Verification items for the finished model (mm, model axes). Face numbers are marked on the shaded views. A direction names the side the tool comes from. Give positions to 0.01 mm unless a question says otherwise; leave off trailing zeros. Loops run counter-clockwise (first coordinate to the right, second up) from the corner with the lowest first, then second, coordinate; pieces in that order, holes last. Notation, with made-up numbers: (-4, 46.5) -> (40, 46.5) arc R21 cw to (40, 60.5) -> close; hole circle Ø4 at (73.5, -23.5). An arc over 180 degrees is marked (long way). Answer in a Markdown table with one row per item. Add a question column.
Q1. Material ranges on probe 1 along Y at (x, z) = (0, 5.3); probe 2 along Y at (x, z) = (-3, -11); probe 3 along Z at (x, y) = (-44.5, 37.5), recorded low to high.
Q2. Gauge pin test, flat ends, axial feed: P1, Ø1, axis at x = -36, z = -14.5, coming from the -Y side; P2, Ø0.6, axis at y = 0.5, z = 5, coming from the +X side; P3, Ø2, axis at x = -12.5, y = -20, coming from the +Z side. Record the tip position at first contact, or that the pin passes through.
Q3. Section check A-A on y = -27.5. Enter the section's corners in (x, z), and give its area (3 significant figures).
Q4. Section check D-D on z = -3.25. Enter the section's corners in (x, y), and give its area (3 significant figures).
Q5. Set-up check for the marked faces 5, 6 and 7: record each of +Z, -Z, +X, -X, +Y, -Y from which the full face is reachable in a straight line by a thin tool's end or side.
Q6. Section check C-C on y = -6. Enter the section's corners in (x, z).
Q7. Release check for a two-part mould opening along Z. For the marked faces 1, 2, 3 and 4 record: pulls with the +Z half, pulls with the -Z half, needs draft (parallel to the pull), parting line crosses it, or undercut.
Q8. Section check B-B on x = -15. Enter the section's corners in (y, z), and give its area (3 significant figures).
```python
from build123d import *

# Parameters (mm, degrees)
EXTRUDE_1_DEPTH     = 4
SKETCH_2_R          = 5
EXTRUDE_2_DEPTH     = 2
SKETCH_3_W          = 0.972791726
SKETCH_3_H          = 7.511993454
EXTRUDE_3_DEPTH     = 2
CUT_EXTRUDE_1_DEPTH = 2
FILLET_1_R          = 2
SKETCH_5_W          = 26
SKETCH_5_H          = 116
EXTRUDE_4_DEPTH     = 14
EXTRUDE_5_DEPTH     = 2


with BuildPart() as part:
    # 草图1 → 凸台-拉伸1 (new body)
    with BuildSketch(Plane.XY):
        with BuildLine():
            Line((-16.5, -55.5), (-16.5, 55.5))
            ThreePointArc((-16.5, 55.5), (0, 72), (16.5, 55.5))
            Line((16.5, 55.5), (16.5, -55.5))
            ThreePointArc((16.5, -55.5), (0, -72), (-16.5, -55.5))
        make_face()
    extrude(amount=EXTRUDE_1_DEPTH)

    # 草图2 → 凸台-拉伸2 (add)
    with BuildSketch(Plane.XY.offset(4)):
        with BuildLine():
            Line((-8.5, -37.5), (-8.5, 37.5))
            ThreePointArc((-8.5, 37.5), (0, 46), (8.5, 37.5))
            Line((8.5, 37.5), (8.5, -37.5))
            ThreePointArc((8.5, -37.5), (0, -46), (-8.5, -37.5))
        make_face()
        with Locations((0, -27.5)):
            Circle(SKETCH_2_R, mode=Mode.SUBTRACT)
    extrude(amount=EXTRUDE_2_DEPTH)

    # 草图3 → 凸台-拉伸3 (add)
    with BuildSketch(Plane.XY.offset(4)):
        with Locations((0, -27.5)):
            Rectangle(SKETCH_3_W, SKETCH_3_H)
    extrude(amount=EXTRUDE_3_DEPTH)

    # 草图4 → 切除-拉伸1 (cut)
    with BuildSketch(Plane.XY.offset(6)):
        Polygon((0, -43.613819341), (4.879446047, -37.404094744), (-5, -37.404094744), align=None)
    extrude(amount=-CUT_EXTRUDE_1_DEPTH, mode=Mode.SUBTRACT)

    # 圆角1
    fillet_1_edges = [part.edges().sort_by_distance(p)[0] for p in [
        (0, -43.613819341, 5),
    ]]
    fillet(fillet_1_edges, radius=FILLET_1_R)

    # 草图5 → 凸台-拉伸4 (add)
    with BuildSketch(Plane(origin=(0, 0, 0), x_dir=(-1, 0, 0), z_dir=(0, 0, -1))):
        Rectangle(SKETCH_5_W, SKETCH_5_H)
    extrude(amount=EXTRUDE_4_DEPTH)

    # 草图6 → 凸台-拉伸5 (add)
    with BuildSketch(Plane(origin=(0, 0, -14), x_dir=(-1, 0, 0), z_dir=(0, 0, -1))):
        with BuildLine():
            Line((0, 58), (67, 58))
            ThreePointArc((67, 58), (70.535533906, 56.535533906), (72, 53))
            Line((72, 53), (72, 38.5))
            ThreePointArc((72, 38.5), (70.535533906, 34.964466094), (67, 33.5))
            Line((67, 33.5), (0, 33.5))
            Line((0, 33.5), (0, 58))
        make_face()
    extrude(amount=EXTRUDE_5_DEPTH)


solid = part.part
```
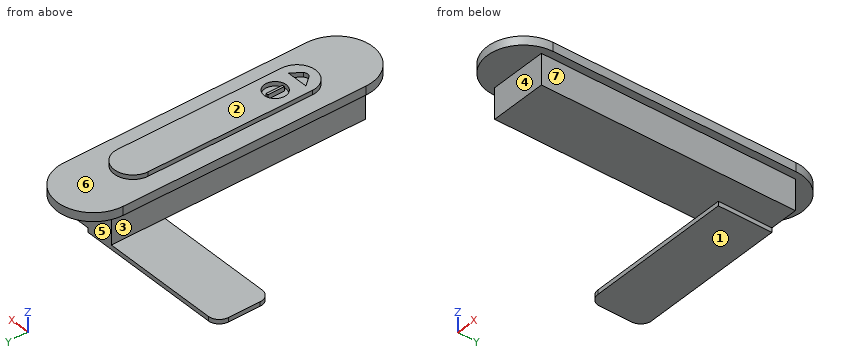
Taken from the geometry:
| question | item | result |
|---|---|---|
| 1 | probe 1 | y = -46 to -42.4, -37.4 to -32.5, -31.26 to -23.74, -22.5 to 46 |
| 1 | probe 2 | y = -58 to 58 |
| 1 | probe 3 | z = -16 to -14 |
| 2 | P1 | stops at y = 33.5 |
| 2 | P2 | stops at x = 8.5 |
| 2 | P3 | stops at z = 4 |
| 3 | outline | (-16.5, 0) -> (-13, 0) -> (-13, -14) -> (13, -14) -> (13, 0) -> (16.5, 0) -> (16.5, 4) -> (8.5, 4) -> (8.5, 6) -> (5, 6) -> (5, 4) -> (0.49, 4) -> (0.49, 6) -> (-0.49, 6) -> (-0.49, 4) -> (-5, 4) -> (-5, 6) -> (-8.5, 6) -> (-8.5, 4) -> (-16.5, 4) -> close |
| 3 | area | 512 mm² |
| 4 | outline | (-13, -58) -> (13, -58) -> (13, 58) -> (-13, 58) -> close |
| 4 | area | 3,020 mm² |
| 5 | face 5 | -Z, +X, -X, +Y |
| 5 | face 6 | +Z |
| 5 | face 7 | -Z, +X, +Y, -Y |
| 6 | outline | (-16.5, 0) -> (-13, 0) -> (-13, -14) -> (13, -14) -> (13, 0) -> (16.5, 0) -> (16.5, 4) -> (8.5, 4) -> (8.5, 6) -> (-8.5, 6) -> (-8.5, 4) -> (-16.5, 4) -> close |
| 7 | face 1 | pulls with the -Z half |
| 7 | face 2 | pulls with the +Z half |
| 7 | face 3 | undercut |
| 7 | face 4 | needs draft |
| 8 | outline | (-62.37, 0) -> (62.37, 0) -> (62.37, 4) -> (-62.37, 4) -> close; (33.5, -16) -> (58, -16) -> (58, -14) -> (33.5, -14) -> close |
| 8 | area | 548 mm² |
